Input: part model. Units: mm. Frame: model coordinates. Face numbers are marked on the shaded views. A direction names the side the tool comes from. Round coordinates to 2 decimals unless told otherwise and drop trailing zeros. Loops run counter-clockwise (first coordinate to the right, second up) from the corner with the lowest first, then second, coordinate; pieces in that order, holes last. Notation, with made-up numbers: M 84,7 L 109,7 A8 cw 109,16 Z; hole C 44.5,-25.75 d10. An arc over 180 degrees is marked long. Return JSON: item names as keys, results as strings. Group by question number.
1) Access query for the marked faces 1, 2 and 3. Directions: +Z, -Z, +X, -X, +Y, -Y. A direction counts if a zero-diameter tool reaches every point of the face in a straight line with its end or side. Return the directions, or none.
2) Mould query, pull axis Z, two halves, no side actions, for the marked faces 4, 5 and 6. Classes: +Z half, -Z half, draft (parallel to the pull), parting line (faces both ways), or undercut.
3) Material intervals for line 1 (Y direction, x = 25, z = 2.8); line 2 (X direction, y = 60, z = 38); line 3 (Z direction, x = 15, y = 23), sorted ascending. Write a range as from..to.
4) Section A-A (y = 15). Count the separate pieces of the cut face and the enclosed holes in it, plus the area to 3 significant figures.
5) Section C-C (x = 25). Output: boundary loops of the cut face in (y, z).
6) Contact query for flat-ended pins moving along their axis: P1, Ø4.5, axis at x = 115, y = 15, coming from the -Z side; P2, Ø1.5, axis at y = 17.5, z = 1.5, coming from the +X side; P3, Ø9, axis at x = 31, z = 16.5, coming from the -Y side; P4, Ø10, axis at x = 67, z = 27, coming from the +Y side. Output: stop coordinate, or through.
7) Section D-D (z = 26.5). Output: boundary loops of the cut face in (x, y), plus the area to 3 significant figures.
Autodesk Inventor part; units mm, degrees
ref_plane "YZ Plane" through (0, 0, 0) normal (1, 0, 0) x (0, 1, 0)
ref_plane "XZ Plane" through (0, 0, 0) normal (0, 1, 0) x (-1, 0, 0)
ref_plane "XY Plane" through (0, 0, 0) normal (0, 0, 1) x (1, 0, 0)
sketch "Sketch1" plane through (0, 0, 0) normal (0, 0, 1) x (1, 0, 0)
  line L0 (0, 0) -> (0, 60)
  arc A0 (50, 60) -> (0, 60) centre (25, 60) ccw
  line L1 (50, 60) -> (50, 30)
  line L2 (50, 30) -> (93.7386, 30)
  line L3 (125.6231, 30) -> (125.6231, 0)
  line L4 (125.6231, 0) -> (0, 0)
  circle A1 centre (25, 60) radius 4.1
  arc A2 (93.7386, 30) -> (68.0182, 121.4364) centre (25, 60) ccw
  arc A3 (125.6231, 30) -> (85.2255, 146.011) centre (25, 60) ccw
  line L5 (68.0182, 121.4364) -> (85.2255, 146.011)
  line L6 (68.0182, 121.4364) -> (25, 60)
  dimension "d0" = 30
  dimension "d1" = 50
  dimension "d2" = 8.2
  dimension "d3" = 30
  dimension "d30" = 55
  dimension "d32" = 30
  dimension "d33" = 75
  dimension "d34" = 105
extrude "Extrusion1" add sketch "Sketch1" along normal blind 5 contours L0 A0 L1 L2 A2 L5 A3 L3 L4
sketch "Sketch2" plane through (0, 0, 5) normal (0, 0, 1) x (1, 0, 0)
  circle A0 centre (25, 15) radius 2.5
  line L0 (0, 0) -> (125.6231, 0)
  line L1 (0, 60) -> (0, 0)
  dimension "d18" = 15
  dimension "d19" = 25
  dimension "d20" = 5
extrude "Extrusion2" cut sketch "Sketch2" against normal blind 10
pattern_linear "Rectangular Pattern1" count 3 spacing 45 along (1, 0, 0) of "Extrusion2"
sketch "Sketch4" plane through (0, 0, 5) normal (0, 0, 1) x (1, 0, 0)
  circle A0 centre (25, 60) radius 4.1
  line L0 (0, 60) -> (0, 0)
  arc A1 (0, 47.3905) -> (32.7178, 33.0847) centre (25, 60) ccw
  line L1 (32.7178, 33.0847) -> (50, 38.0403)
  line L2 (50, 30) -> (50, 60)
  line L3 (0, 47.3905) -> (0, 30)
  line L4 (93.7386, 30) -> (50, 30)
  line L5 (0, 30) -> (50, 30)
  line L6 (50, 30) -> (50, 38.0403)
  dimension "d26" = 28
  dimension "d27" = 16
extrude "Extrusion3" add sketch "Sketch4" along normal blind 15 contours A1 L1 L2 L5 L0
sketch "Sketch5" plane through (0, 0, 5) normal (0, 0, 1) x (1, 0, 0)
  circle A0 centre (25, 60) radius 4.1
  arc A1 (100.7286, 80.2914) -> (80.4372, 115.4372) centre (25, 60) ccw
  arc A2 (103.8195, 81.1196) -> (82.6999, 117.6999) centre (25, 60) ccw
  arc A3 (120.0471, 85.4678) -> (94.5793, 129.5793) centre (25, 60) ccw
  arc A4 (123.1381, 86.296) -> (96.842, 131.842) centre (25, 60) ccw
  arc A5 (82.6999, 117.6999) -> (80.4372, 115.4372) centre (81.5685, 116.5685) ccw
  arc A6 (100.7286, 80.2914) -> (103.8195, 81.1196) centre (102.2741, 80.7055) ccw
  arc A7 (96.842, 131.842) -> (94.5793, 129.5793) centre (95.7107, 130.7107) ccw
  arc A8 (120.0471, 85.4678) -> (123.1381, 86.296) centre (121.5926, 85.8819) ccw
  line L0 (95.7107, 130.7107) -> (81.5685, 116.5685)
  line L1 (81.5685, 116.5685) -> (25, 60)
  line L2 (25, 60) -> (102.2741, 80.7055)
  line L3 (102.2741, 80.7055) -> (121.5926, 85.8819)
  line L4 (93.7386, 30) -> (50, 30)
  point P0 (0, 0)
  dimension "d35" = 3.2
  dimension "d36" = 3.2
  dimension "d37" = 45
  dimension "d38" = 15
  dimension "d44" = 80
  dimension "d45" = 20
extrude "Extrusion4" cut sketch "Sketch5" against normal blind 15 contours L2 L3 A6 | A1 L1 L0 A2 L3 L2 | A5 L0 L1 | A3 A7 A4 A8
sketch "Sketch6" plane through (0, 0, 5) normal (0, 0, 1) x (1, 0, 0)
  circle A0 centre (25, 60) radius 4.1
  arc A1 (125.6231, 30) -> (85.2255, 146.011) centre (25, 60) ccw
  arc A2 (125.6231, 30) -> (129.9954, 60.9786) centre (25, 60) ccw
  arc A3 (93.7386, 30) -> (68.0182, 121.4364) centre (25, 60) ccw
  arc A4 (93.7386, 30) -> (99.5998, 52.2628) centre (25, 60) ccw
  line L0 (99.5998, 52.2628) -> (129.9954, 60.9786)
  line L1 (93.7386, 30) -> (125.6231, 30)
  line L2 (50, 38.0403) -> (32.7178, 33.0847)
  point P0 (0, 0)
extrude "Extrusion5" add sketch "Sketch6" along normal blind 15 contours L1 A3 L0 A1
mirror "Mirror1" about plane through (111.8693, 45.4893, 20) normal (0, 0, 1)
sketch "Sketch7" plane through (68.0182, 121.4364, 0) normal (-0.8192, 0.5736, 0) x (0, 0, 1)
  line L0 (0, -41.8595) -> (0, 30)
  line L1 (40, 30) -> (35, 30)
  line L2 (0, 0) -> (40, 0)
  line L3 (40, 0) -> (40, 30)
  line L4 (40, 30) -> (0, 30)
  line L5 (0, 30) -> (0, 0)
  point P0 (0, -138.4885)
  point P1 (35, 30)
  point P2 (0, 30)
extrude "Extrusion6" add sketch "Sketch7" along normal blind 7
properties part number "force_measurement_plate"
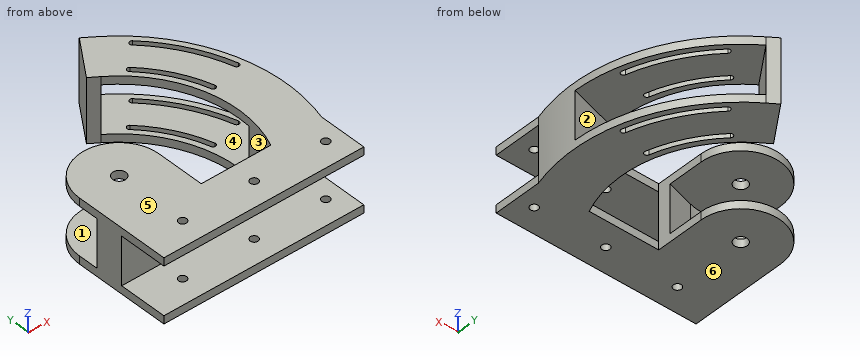
Returned:
{
 "1": {"face 1": "+Y", "face 2": "-X, +Y", "face 3": "+Z, -Z"},
 "2": {"face 4": "undercut", "face 5": "+Z half", "face 6": "-Z half"},
 "3": {"line 1": "y = 0..12.5, 17.5..55.9, 64.1..85", "line 2": "x = 0..20.9, 29.1..50, 100..130", "line 3": "z = 0..5, 35..40"},
 "4": {"separate pieces": "8", "enclosed holes": "0", "area": "1,110 mm^2"},
 "5": {"outline": "M 0,0 L 12.5,0 L 12.5,5 L 0,5 Z; M 0,35 L 12.5,35 L 12.5,40 L 0,40 Z; M 17.5,0 L 55.9,0 L 55.9,5 L 32,5 L 32,35 L 55.9,35 L 55.9,40 L 17.5,40 L 17.5,35 L 30,35 L 30,5 L 17.5,5 Z; M 64.1,0 L 85,0 L 85,5 L 64.1,5 Z; M 64.1,35 L 85,35 L 85,40 L 64.1,40 Z"},
 "6": {"P1": "passes through", "P2": "stops at x = 125.62", "P3": "stops at y = 30", "P4": "stops at y = 139.33"},
 "7": {"outline": "M 0,30 L 50,30 L 50,38.04 L 32.72,33.08 A28 cw 0,47.39 Z; M 62.28,125.45 L 68.02,121.44 L 85.23,146.01 L 79.49,150.03 Z; M 93.74,30 L 125.62,30 A105 ccw 130,60.98 L 99.6,52.26 A75 cw Z", "area": "1,300 mm^2"}
}
